Model file for the job. Use its own axes, mm. A direction names the side the tool comes from. Give positions to 0.01 mm unless a question says otherwise; leave off trailing zeros. Loops run counter-clockwise (first coordinate to the right, second up) from the corner with the lowest first, then second, coordinate; pieces in that order, holes last. Notation, with made-up numbers: M 46,-9 L 86,-9 A15 ccw 86,8 Z; hole C -32.5,16 d5. An arc over 180 degrees is marked long. Answer in a Markdown table with one row per item.
```python
from build123d import *

# Parameters (mm, degrees)
F0_W     = 85.1905047894
F0_H     = 132.3906481266
F0_W_2   = 70.8002224565
F0_H_2   = 118.5759752989
F1_DEPTH = 88.392
F2_W     = 62.7876967192
F2_H     = 41.029587388
F3_DEPTH = 85.1915047894
F4_DEPTH = 10.922
F5_R     = 8.4882818578
F6_DEPTH = 132.3916481266


with BuildPart() as f1:
    # F0 (on Top) → F1 (new body)
    with BuildSketch(Plane.XY):
        Rectangle(F0_W, F0_H)
        Rectangle(F0_W_2, F0_H_2, mode=Mode.SUBTRACT)
    extrude(amount=F1_DEPTH)

    # F2 (on face) → F3 (cut, through all)
    with BuildSketch(Plane(origin=(-42.5952523947, 0, 0), x_dir=(0, -1, 0), z_dir=(-1, 0, 0))):
        with Locations((0, 67.6403790712)):
            Rectangle(F2_W, F2_H)
    extrude(amount=-F3_DEPTH, mode=Mode.SUBTRACT)

    # F4 (cut): a face of the model
    f4_faces = [f1.faces().sort_by_distance(p)[0] for p in [
        (0, -64.6210081542, 88.392),
    ]]
    extrude(f4_faces, amount=-F4_DEPTH, mode=Mode.SUBTRACT)

    # F5 (on face) → F6 (cut, through all)
    with BuildSketch(Plane.XZ.offset(66.1953240633)):
        with Locations((0, 41.9554561377)):
            Circle(F5_R)
    extrude(amount=-F6_DEPTH, mode=Mode.SUBTRACT)


solid = f1.part
```
(1) Saw through at B-B, the plane x = 0. Give the cut face in (y, z), and give its area (3 significant figures).
Established:
| item | result |
|---|---|
| outline | M -66.2,0 L -59.29,0 L -59.29,33.47 L -66.2,33.47 Z; M -66.2,50.44 L -59.29,50.44 L -59.29,77.47 L -66.2,77.47 Z; M 59.29,0 L 66.2,0 L 66.2,33.47 L 59.29,33.47 Z; M 59.29,50.44 L 66.2,50.44 L 66.2,77.47 L 59.29,77.47 Z |
| area | 836 mm2 |
(2) Saw through at C-C, the plane z = 22. Give the cut face in (x, y).
Established:
| item | result |
|---|---|
| outline | M -42.6,-66.2 L 42.6,-66.2 L 42.6,66.2 L -42.6,66.2 Z; hole M -35.4,-59.29 L 35.4,-59.29 L 35.4,59.29 L -35.4,59.29 Z |
(3) Which spindle directions (+Z, -Z, +X, -X, +Y, -Y) get a long thin tool onto all of the face, cutting with end or side? Do faces 4 (the flat face through (35.4, -1, 30)), 5 (the flat face through (-39, -31.394, 62)), 6 (the flat face through (-1, -66.195, 30)). Say none if no direction does.
Established:
| item | result |
|---|---|
| face 4 | +Z, -Z |
| face 5 | +Z, +X, -X |
| face 6 | +Z, -Z, +X, -X, -Y |
(4) Mould opens along Z. For faces 1 (the flat face through (-38, 5, 0)), 2 (the cylindrical face through (4.563, 62.693, 49.113)), 3 (the flat face through (39, -31.394, 62)) say: pulls with the +Z half, pulls with the -Z half, needs draft (parallel to the pull), parting line crosses it, or undercut.
Established:
| item | result |
|---|---|
| face 1 | pulls with the -Z half |
| face 2 | undercut |
| face 3 | needs draft |
(5) Saw through at D-D, the plane z = 37.5. Give the cut face in (x, y).
Established:
| item | result |
|---|---|
| outline | M -42.6,-66.2 L -7.22,-66.2 L -7.22,-59.29 L -35.4,-59.29 L -35.4,59.29 L -7.22,59.29 L -7.22,66.2 L -42.6,66.2 Z; M 7.22,-66.2 L 42.6,-66.2 L 42.6,66.2 L 7.22,66.2 L 7.22,59.29 L 35.4,59.29 L 35.4,-59.29 L 7.22,-59.29 Z |
(6) Flat gauge pins, fed straight in: P1, Ø13.5, axis at x = 0, z = 41.96, coming from the +Y side; P2, Ø8, axis at x = 40, y = -11, coming from the +Z side. Where does each tip first touch, or does it go through?
Established:
| item | result |
|---|---|
| P1 | passes through |
| P2 | stops at z = 47.13 |
(7) Wall check: L1, parallel to Y at x = -9, z = 35.5; L2, parallel to X at y = 34, z = 74; L3, parallel to Z at x = 0, y = 61. Give the ranges that are in metal, low to high.
Established:
| item | result |
|---|---|
| L1 | y = -66.2 to -59.29, 59.29 to 66.2 |
| L2 | x = -42.6 to -35.4, 35.4 to 42.6 |
| L3 | z = 0 to 33.47, 50.44 to 77.47 |
(8) Saw through at A-A, the plane y = 52.5. Give the cut face in (x, z).
Established:
| item | result |
|---|---|
| outline | M -42.6,0 L -35.4,0 L -35.4,77.47 L -42.6,77.47 Z; M 35.4,0 L 42.6,0 L 42.6,77.47 L 35.4,77.47 Z |
